Autodesk Inventor part; units mm, degrees
ref_plane "Arbeitsebene1" through (-9, -9, -7.8) normal (0, 0, -1) x (0, 1, 0)
ref_plane "YZ Plane" through (0, 0, 0) normal (1, 0, 0) x (0, 1, 0)
ref_plane "XZ Plane" through (0, 0, 0) normal (0, 1, 0) x (-1, 0, 0)
sketch "Skizze1" plane through (0, 0, 0) normal (0, 0, 1) x (1, 0, 0)
  arc A0 (-9, -8) -> (-8, -9) centre (-8, -8) ccw
  line L0 (8, -9) -> (-8, -9)
  arc A1 (8, -9) -> (9, -8) centre (8, -8) ccw
  line L1 (9, 8) -> (9, -8)
  arc A2 (9, 8) -> (8, 9) centre (8, 8) ccw
  line L2 (-8, 9) -> (8, 9)
  arc A3 (-8, 9) -> (-9, 8) centre (-8, 8) ccw
  line L3 (-9, -8) -> (-9, 8)
  circle A4 centre (0, 0) radius 5.8
  arc A5 (-8, 9.1) -> (-9.1, 8) centre (-8, 8) ccw
  line L4 (-8, 9.1) -> (8, 9.1)
  arc A6 (9.1, 8) -> (8, 9.1) centre (8, 8) ccw
  line L5 (9.1, 8) -> (9.1, -8)
  arc A7 (8, -9.1) -> (9.1, -8) centre (8, -8) ccw
  line L6 (8, -9.1) -> (-8, -9.1)
  arc A8 (-9.1, -8) -> (-8, -9.1) centre (-8, -8) ccw
  line L7 (-9.1, -8) -> (-9.1, 8)
  line L8 (14, 14) -> (-14, 14)
  line L9 (-14, 14) -> (-14, -14)
  line L10 (-14, -14) -> (14, -14)
  line L11 (14, -14) -> (14, 14)
  line L12 (14, 14) -> (-14, -14) construction
  line L13 (-14, 14) -> (14, -14) construction
  point P0 (0, 0)
  dimension "d0" = 0.1
  dimension "d1" = 28
  dimension "d2" = 28
ref_plane "Arbeitsebene1" through (-9, -9, -7.8) normal (0, 0, -1) x (0, 1, 0)
extrude "Extrusion1" add sketch "Skizze1" against normal up to surface (7.8 mm away) contours L11 L10 L9 L8
sketch "Skizze2" plane through (0, 0, 0) normal (0, 0, 1) x (1, 0, 0)
  line L0 (-14, 14) -> (-14, -14)
  line L1 (-14, -14) -> (14, -14)
  line L2 (14, -14) -> (14, 14)
  line L3 (14, 14) -> (-14, 14)
  line L4 (9.1, 8) -> (9.1, -8)
  arc A0 (8, -9.1) -> (9.1, -8) centre (8, -8) ccw
  line L5 (8, -9.1) -> (-8, -9.1)
  arc A1 (-9.1, -8) -> (-8, -9.1) centre (-8, -8) ccw
  line L6 (-9.1, -8) -> (-9.1, 8)
  arc A2 (-8, 9.1) -> (-9.1, 8) centre (-8, 8) ccw
  line L7 (-8, 9.1) -> (8, 9.1)
  arc A3 (9.1, 8) -> (8, 9.1) centre (8, 8) ccw
  line L8 (-7.6, 7.6) -> (-7.6, -7.6)
  line L9 (-7.6, -7.6) -> (7.6, -7.6)
  line L10 (7.6, -7.6) -> (7.6, 7.6)
  line L11 (7.6, 7.6) -> (-7.6, 7.6)
  point P0 (0, 0)
  dimension "d5" = 1.5
extrude "Extrusion2" add sketch "Skizze2" along normal blind 0.5 contours L3 L2 L1 L0 | L4 A0 L5 A1 L6 A2 L7 A3 | L11 L10 L9 L8
sketch "Skizze3" plane through (0, 0, 0.5) normal (0, 0, 1) x (1, 0, 0)
  line L0 (-14, -14) -> (14, -14)
  line L1 (14, -14) -> (14, 14)
  line L2 (14, 14) -> (-14, 14)
  line L3 (-14, 14) -> (-14, -14)
  circle A0 centre (0, 4.2) radius 4
  circle A1 centre (-9, -3.3) radius 2
  circle A2 centre (-9, 11.7) radius 2
  line L4 (-15, 21.2) -> (-15, 16.05)
  line L5 (-15, 16.05) -> (-12, 16.05)
  line L6 (-12, 16.05) -> (-12, 13.55)
  line L7 (-12, 13.55) -> (-15, 13.55)
  line L8 (-15, 13.55) -> (-15, 1.15)
  line L9 (-15, 1.15) -> (-12, 1.15)
  line L10 (-12, 1.15) -> (-12, -1.35)
  line L11 (-12, -1.35) -> (-15, -1.35)
  line L12 (-15, -1.35) -> (-15, -5.8)
  line L13 (-15, -5.8) -> (0, -5.8)
  line L14 (0, -5.8) -> (0, 0.2)
  arc A3 (0, 8.2) -> (0, 0.2) centre (0, 4.2) ccw
  line L15 (0, 8.2) -> (0, 21.2)
  line L16 (-15, 21.2) -> (0, 21.2)
  dimension "d8" = 8
extrude "Extrusion3" add sketch "Skizze3" along normal blind 3 contours L3 L13 L14 A0 L15 L2 L1 L0 | L3 L11 L10 L9 L7 L6 L2 L15 A0 L14 L13 | L3 L9 L10 L11 | L6 L7 L3 L2 | A1 | A2
sketch "Skizze4" plane through (0, 0, 3.5) normal (0, 0, 1) x (1, 0, 0)
  line L0 (14, -14) -> (14, 14)
  line L1 (14, 14) -> (-14, 14)
  line L2 (-14, 14) -> (-14, -14)
  line L3 (-14, -14) -> (14, -14)
  circle A0 centre (0, 4.2) radius 4
  line L4 (5, -10.8) -> (-5, -10.8)
  line L5 (-14, 14) -> (-14, -14)
  line L6 (14, -14) -> (-14, -14)
  line L7 (-14, -14) -> (-14, -9.3)
  line L8 (-14, -9.3) -> (14, -9.3)
  line L9 (14, -9.3) -> (14, -14)
  line L10 (-14, 14) -> (-12.5, 14)
  line L11 (-12.5, 14) -> (-12.5, -9.3)
  line L12 (-12.5, -9.3) -> (-14, -9.3)
  line L13 (-14, -9.3) -> (-14, 14)
  line L14 (14, -14) -> (14, 14)
  line L15 (14, 14) -> (12.5, 14)
  line L16 (12.5, 14) -> (12.5, -9.3)
  line L17 (12.5, -9.3) -> (14, -9.3)
  line L18 (14, -9.3) -> (14, 14)
  point P0 (0, 0)
  point P1 (14, -9.3)
  point P2 (12.5, 14)
  dimension "d11" = 1.5
  dimension "d22" = 1.5
  dimension "d23" = 1.5
extrude "Extrusion4" cut sketch "Skizze4" against normal through all contours L3 L2 L8 L0 | L8 L16 L1 L0 | L2 L1 L11 L8
sketch "Skizze5" plane through (0, 0, 3.5) normal (0, 0, 1) x (1, 0, 0)
  circle A0 centre (-9, 11.7) radius 2
  circle A1 centre (-9, -3.3) radius 2.5019
  line L0 (-9, -3.3) -> (9, -3.3)
  line L1 (9, -3.3) -> (9, 11.7)
  line L2 (9, 11.7) -> (-9, 11.7)
  line L3 (-9, 11.7) -> (-9, -3.3)
  dimension "d25" = 18
hole "Bohrung1" at (9, -3.3, 3.5) at (9, 11.7, 3.5) at (-9, -3.3, 3.5) at (-9, 11.7, 3.5) direction (0, 0, -1) diameter 3 depth 0.0001 tip angle 140
properties part number "10_SOOCT_VCM_Mount_v3"
Build history of the part. All positions in model axes, mm. A direction names the side the tool comes from. Round coordinates to 2 decimals unless told otherwise and drop trailing zeros. Loops run counter-clockwise (first coordinate to the right, second up) from the corner with the lowest first, then second, coordinate; pieces in that order, holes last. Notation, with made-up numbers: (-31, -22) -> (-11, -22) arc R22 cw to (-11, -15) -> close; hole circle Ø4 at (29, -26.5). An arc over 180 degrees is marked (long way). Use CSV: the item, a comma, the result in double quotes. Start each with the question number.
Q1. Saw through at A-A on x = -6. Give the cut face in (y, z).
Q2. Mould opens along Y. For faces 1 (the face through (0, 0, 3.5)), 2 (the face through (0, 14, -2)), 3 (the face through (8.786, 8.769, -3.845)) say: +Y half, -Y half, draft (parallel to the pull), parting line (faces both ways), or undercut.
Q3. Which spindle directions (+Z, -Z, +X, -X, +Y, -Y) get a long thin tool onto all of the face, cutting with end or side? Do faces 4 (the face through (-9.1, 0, -4)), 5 (the face through (-0.867, 8.105, 1.979)), 6 (the face through (12.5, 3, -2)). Say none if no direction does.
Q4. Saw through at B-B on y = 4.2. Give the cut face in (x, z), and give its area (3 significant figures).
Q5. Saw through at C-C on z = -4.75. Give the cut face in (x, y), and give its area (3 significant figures).
Q6. Drill centre lines: L1, parallel to X at y = -1.5, z = -5; L2, parallel to Y at x = 7.5, z = -5.75; L3, parallel to Z at x = 3.5, y = -6.25. Where is each one in solid material? Low to high.
Q7. Flat gauge pins, fed straight in: pin 1 Ø9 at (x, y) = (-3, -1.5) entering from -Z; pin 2 Ø2 at (x, y) = (9, -6.5) entering from -Z; pin 3 Ø4 at (x, y) = (0.5, 6) entering from +Z. Where does each tip first touch, or does it go through?
Q8. Saw through at D-D on x = 0. Give the cut face in (y, z).
Solutions:
1,outline,"(-9.3, -7.8) -> (-9.1, -7.8) -> (-9.1, 0) -> (9.1, 0) -> (9.1, -7.8) -> (14, -7.8) -> (14, 3.5) -> (-9.3, 3.5) -> close"
2,face 1,"draft"
2,face 2,"+Y half"
2,face 3,"undercut"
3,face 4,"-Z"
3,face 5,"+Z"
3,face 6,"+Z, -Z, +X, +Y, -Y"
4,outline,"(-12.5, -7.8) -> (-9.1, -7.8) -> (-9.1, 0) -> (9.1, 0) -> (9.1, -7.8) -> (12.5, -7.8) -> (12.5, 3.5) -> (4, 3.5) -> (4, 0.5) -> (-4, 0.5) -> (-4, 3.5) -> (-12.5, 3.5) -> close"
4,area,"117 mm^2"
5,outline,"(-12.5, -9.3) -> (12.5, -9.3) -> (12.5, 14) -> (-12.5, 14) -> close; hole (-9.1, -8) arc R1.1 ccw to (-8, -9.1) -> (8, -9.1) arc R1.1 ccw to (9.1, -8) -> (9.1, 8) arc R1.1 ccw to (8, 9.1) -> (-8, 9.1) arc R1.1 ccw to (-9.1, 8) -> close"
5,area,"252 mm^2"
6,L1,"x = -12.5 to -9.1, 9.1 to 12.5"
6,L2,"y = -9.3 to -9.1, 9.1 to 14"
6,L3,"z = 0 to 3.5"
7,pin 1,"stops at z = 0"
7,pin 2,"stops at z = -7.8"
7,pin 3,"stops at z = 0.5"
8,outline,"(-9.3, -7.8) -> (-9.1, -7.8) -> (-9.1, 0) -> (9.1, 0) -> (9.1, -7.8) -> (14, -7.8) -> (14, 3.5) -> (8.2, 3.5) -> (8.2, 0.5) -> (0.2, 0.5) -> (0.2, 3.5) -> (-9.3, 3.5) -> close"
